```python
from build123d import *

# Parameters (mm, degrees)
SKETCH1_W           = 12.7
SKETCH1_H           = 38.1
BOSS_EXTRUDE1_DEPTH = 155.575
SKETCH3_W           = 12.7
SKETCH3_H           = 38.1
BOSS_EXTRUDE2_DEPTH = 130.175
SKETCH4_W           = 100.6348
SKETCH4_H           = 12.192
BOSS_EXTRUDE3_DEPTH = 101.0412
CUT_EXTRUDE2_DEPTH  = 12.192
BOSS_EXTRUDE8_START = -60.96
SKETCH6_R           = 44.45
SKETCH6_R_2         = 39.3192
BOSS_EXTRUDE8_DEPTH = 60.96


with BuildPart() as part:
    # Sketch1 → Boss-Extrude1 (new body)
    with BuildSketch(Plane(origin=(0, 0, 0), x_dir=(0, -1, 0), z_dir=(-1, 0, 0))):
        with Locations((-6.35, 19.05)):
            Rectangle(SKETCH1_W, SKETCH1_H)
    extrude(amount=-BOSS_EXTRUDE1_DEPTH)

    # Sketch3 → Boss-Extrude2 (add)
    with BuildSketch(Plane(origin=(0, 12.7, 0), x_dir=(1, 0, 0), z_dir=(0, 1, 0))):
        with Locations((6.35, -19.05)):
            Rectangle(SKETCH3_W, SKETCH3_H)
    extrude(amount=BOSS_EXTRUDE2_DEPTH)

    # Sketch4 → Boss-Extrude3 (add)
    with BuildSketch(Plane(origin=(0, 12.7, 0), x_dir=(1, 0, 0), z_dir=(0, 1, 0))):
        with Locations((63.0174, -18.796)):
            Rectangle(SKETCH4_W, SKETCH4_H)
    extrude(amount=BOSS_EXTRUDE3_DEPTH)

    # Sketch5 → Cut-Extrude2 (cut)
    with BuildSketch(Plane.XY.offset(24.892)):
        Polygon((12.7, 58.42), (58.42, 12.7), (12.7, 12.7), align=None)
    extrude(amount=-CUT_EXTRUDE2_DEPTH, mode=Mode.SUBTRACT)

    # Sketch6 → Boss-Extrude8 (add)
    with BuildSketch(Plane(origin=(0, 0, 24.892), x_dir=(-1, 0, 0), z_dir=(0, 0, -1)).offset(BOSS_EXTRUDE8_START)):
        with Locations(Location((-57.2008, 57.2008, 0), (0, 0, 180))):
            Circle(SKETCH6_R)
        with Locations(Location((-57.2008, 57.2008, 0), (0, 0, 180))):
            Circle(SKETCH6_R_2, mode=Mode.SUBTRACT)
    extrude(amount=BOSS_EXTRUDE8_DEPTH)


solid = part.part
```
Source: CAD feature listing. Evaluate the final solid. Frame: model axes, mm. A direction names the side the tool comes from. Round coordinates to 2 decimals unless told otherwise and drop trailing zeros. Write each loop counter-clockwise with the first axis right and the second up, starting at its lowest first coordinate (ties: lowest second). Pieces come first, ordered by that corner, then holes. Notation, with made-up numbers: M 51,46.25 L 105,46.25 A23 cw 105,83.25 Z; hole C 52.5,-11 d5. An arc over 180 degrees is marked long. Use CSV: the item, a comma, the result in double quotes. Start each with the question number.
Q1. First-contact query: P1, Ø23.5, axis at x = 54.5, y = 54, coming from the +Z side; P2, Ø10, axis at y = 72, z = 20, coming from the +X side; P3, Ø10, axis at x = 54, z = 22.5, coming from the -Y side; P4, Ø12, axis at y = 89, z = 51, coming from the +X side. Flat tips, straight axial feed; report the tip coordinate or a pass-through.
Q2. Access query for faces 5 (the face through (62, 63, 12.7)), 6 (the face through (43, 8, 38.1)), 7 (the face through (57, 57, 24.892)), 8 (the face through (29, 29, 24.892)). Directions: +Z, -Z, +X, -X, +Y, -Y. A direction counts if a zero-diameter tool reaches every point of the face in a straight line with its end or side. Return the directions, or none.
Q3. Pull-direction query (Y, two-part tool) for faces 1 (the face through (113.335, 63, 19)), 2 (the face through (62, 113.741, 19)), 3 (the face through (83, 12.7, 27)), 4 (the face through (77, 0, 19)); classes: +Y half, -Y half, draft (parallel to the pull), parting line (faces both ways), or undercut.
Q4. Cut plane B-B on y = 22. Output: boundary loops of the cut face in (x, z).
Q5. Cut plane C-C on x = 31. Output: boundary loops of the cut face in (y, z), plus the area to 3 significant figures.
Q6. Line query: line 1 (Y direction, x = 86.5, z = 38); line 2 (Y direction, x = 62, z = 25.5); line 3 (X direction, y = 75.5, z = 14). Output: solid intervals per line, ascending. Write a range as from..to.
Q7. Cut plane D-D on y = 55. Output: boundary loops of the cut face in (x, z).
Q8. Cut plane A-A on z = 28.5. Output: boundary loops of the cut face in (x, y) (3 decimals).
Results found:
1,P1,"z = 24.89"
1,P2,"x = 113.33"
1,P3,"y = 0"
1,P4,"x = 93.4"
2,face 5,"-Z, +X, +Y"
2,face 6,"+Z, -X, -Y"
2,face 7,"+Z"
2,face 8,"-Z"
3,face 1,"draft"
3,face 2,"+Y half"
3,face 3,"undercut"
3,face 4,"-Y half"
4,outline,"M 0,0 L 12.7,0 L 12.7,38.1 L 0,38.1 Z; M 30.06,24.89 L 39.68,24.89 L 39.68,85.85 L 30.06,85.85 Z; M 49.12,12.7 L 113.33,12.7 L 113.33,24.89 L 84.34,24.89 L 84.34,85.85 L 74.72,85.85 L 74.72,24.89 L 49.12,24.89 Z"
5,outline,"M 0,0 L 12.7,0 L 12.7,38.1 L 0,38.1 Z; M 21.29,24.89 L 27.88,24.89 L 27.88,85.85 L 21.29,85.85 Z; M 40.12,12.7 L 113.74,12.7 L 113.74,24.89 L 93.11,24.89 L 93.11,85.85 L 86.52,85.85 L 86.52,24.89 L 40.12,24.89 Z"
5,area,"2,180 mm^2"
6,line 1,"0..12.7, 23.77..30.98, 83.42..90.63"
6,line 2,"0..12.7, 13.01..18.18, 96.23..101.39"
6,line 3,"0..113.33"
7,outline,"M 0,0 L 12.7,0 L 12.7,38.1 L 0,38.1 Z; M 12.81,24.89 L 16.12,24.89 L 16.12,12.7 L 113.33,12.7 L 113.33,24.89 L 101.6,24.89 L 101.6,85.85 L 96.46,85.85 L 96.46,24.89 L 17.94,24.89 L 17.94,85.85 L 12.81,85.85 Z"
8,outline,"M 0,0 L 155.575,0 L 155.575,12.7 L 12.7,12.7 L 12.7,142.875 L 0,142.875 Z; C 57.201,57.201 d88.9; hole C 57.201,57.201 d78.638"
